from build123d import *

# Parameters (mm, degrees)
SKETCH1_W           = 609.6
SKETCH1_H           = 609.6
BOSS_EXTRUDE1_DEPTH = 6.35
CUT_EXTRUDE2_DEPTH  = 432.099063441
SKETCH4_W           = 25.4
SKETCH4_H           = 25.4
CUT_EXTRUDE8_DEPTH  = 432.099063441
FILLET4_R           = 12.7
FILLET5_R           = 12.7
SKETCH5_R           = 3.175
CUT_EXTRUDE9_DEPTH  = 432.099063441
FILLET9_R           = 1.5875


with BuildPart() as part:
    # Sketch1 → Boss-Extrude1 (new body)
    with BuildSketch(Plane(origin=(0, 0, 0), x_dir=(1, 0, 0), z_dir=(0, 1, 0))):
        Rectangle(SKETCH1_W, SKETCH1_H)
    extrude(amount=BOSS_EXTRUDE1_DEPTH)

    # Sketch3 → Cut-Extrude2 (cut, through all)
    with BuildSketch(Plane(origin=(0, 0, 0), x_dir=(1, 0, 0), z_dir=(0, 1, 0))):
        with BuildLine():
            Line((-3.175, 248.4755), (-3.175, 142.454689298))
            ThreePointArc((-3.175, 142.454689298), (-45.125573361, 120.304111538), (-50.492310608, 73.169232396))
            ThreePointArc((-50.492310608, 73.169232396), (-76.989658396, 44.45), (-88.612569335, 7.143007484))
            ThreePointArc((-88.612569335, 7.143007484), (-126.749203452, -21.072162878), (-124.95687982, -68.477713992))
            Line((-124.95687982, -68.477713992), (-216.773595218, -121.488119343))
            Line((-216.773595218, -121.488119343), (-213.598595218, -126.987380657))
            Line((-213.598595218, -126.987380657), (-121.78187982, -73.976975306))
            ThreePointArc((-121.78187982, -73.976975306), (-81.623630091, -99.23194866), (-38.120258727, -80.31223988))
            ThreePointArc((-38.120258727, -80.31223988), (0, -88.9), (38.120258727, -80.31223988))
            ThreePointArc((38.120258727, -80.31223988), (81.623630091, -99.23194866), (121.78187982, -73.976975306))
            Line((121.78187982, -73.976975306), (213.598595218, -126.987380657))
            Line((213.598595218, -126.987380657), (216.773595218, -121.488119343))
            Line((216.773595218, -121.488119343), (124.95687982, -68.477713992))
            ThreePointArc((124.95687982, -68.477713992), (126.749203452, -21.072162878), (88.612569335, 7.143007484))
            ThreePointArc((88.612569335, 7.143007484), (76.989658396, 44.45), (50.492310608, 73.169232396))
            ThreePointArc((50.492310608, 73.169232396), (45.125573361, 120.304111538), (3.175, 142.454689298))
            Line((3.175, 142.454689298), (3.175, 248.4755))
            Line((3.175, 248.4755), (-3.175, 248.4755))
        make_face()
    extrude(amount=CUT_EXTRUDE2_DEPTH, mode=Mode.SUBTRACT)

    # Sketch4 → Cut-Extrude8 (cut, through all)
    with BuildSketch(Plane(origin=(0, 0, 0), x_dir=(1, 0, 0), z_dir=(0, 1, 0))):
        with Locations((12.7, -190.5)):
            Rectangle(SKETCH4_W, SKETCH4_H)
        with Locations((-190.5, 12.7)):
            Rectangle(SKETCH4_W, SKETCH4_H)
    extrude(amount=CUT_EXTRUDE8_DEPTH, mode=Mode.SUBTRACT)

    # Fillet4
    fillet4_edges = [part.edges().sort_by_distance(p)[0] for p in [
        (-177.8, 3.175, -25.4),
    ]]
    fillet(fillet4_edges, radius=FILLET4_R)

    # Fillet5
    fillet5_edges = [part.edges().sort_by_distance(p)[0] for p in [
        (25.4, 3.175, 177.8),
    ]]
    fillet(fillet5_edges, radius=FILLET5_R)

    # Sketch5 → Cut-Extrude9 (cut, through all)
    with BuildSketch(Plane(origin=(0, 6.35, 0), x_dir=(1, 0, 0), z_dir=(0, 1, 0))):
        with Locations(Location((-254, 254, 0), (0, 0, 270))):
            Circle(SKETCH5_R)
        with Locations(Location((254, 254, 0), (0, 0, 270))):
            Circle(SKETCH5_R)
        with Locations(Location((254, -254, 0), (0, 0, 270))):
            Circle(SKETCH5_R)
        with Locations(Location((-254, -254, 0), (0, 0, 270))):
            Circle(SKETCH5_R)
    extrude(amount=-CUT_EXTRUDE9_DEPTH, mode=Mode.SUBTRACT)

    # Fillet9
    fillet9_edges = [part.edges().sort_by_distance(p)[0] for p in [
        (3.175, 3.175, -248.4755),
        (-3.175, 3.175, -248.4755),
        (-216.773595218, 3.175, 121.488119343),
        (-213.598595218, 3.175, 126.987380657),
        (213.598595218, 3.175, 126.987380657),
        (216.773595218, 3.175, 121.488119343),
    ]]
    fillet(fillet9_edges, radius=FILLET9_R)


solid = part.part
Check sheet for the modelled part. Datum: model origin and axes. Units: mm. A direction names the side the tool comes from. Round coordinates to 2 decimals unless told otherwise and drop trailing zeros. Loops run counter-clockwise (first coordinate to the right, second up) from the corner with the lowest first, then second, coordinate; pieces in that order, holes last. Notation, with made-up numbers: M 18,51 L 65,51 A33 cw 65,80 Z; hole C -40,40.25 d7. An arc over 180 degrees is marked long. One line per item, written item: value.
(1) Sectioned sample at A-A, the plane z = -66. Record the cut outline in (x, y), then the cut area to 3 significant figures.
Computed values:
outline: M -304.8,0 L -59.56,0 L -59.56,6.35 L -304.8,6.35 Z; M 59.56,0 L 304.8,0 L 304.8,6.35 L 59.56,6.35 Z
area: 3,110 mm^2
(2) Access from +Z, -Z, +X, -X, +Y, -Y to the whole of each face (thin tool, end or side, straight path). Record for faces 1 (the face through (166.37, 3.13, 99.72)), 2 (the face through (63, 6.35, -72)).
Computed values:
face 1: +Y, -Y
face 2: +Z, -Z, +X, -X, +Y
(3) Sectioned sample at B-B, the plane x = 106. Record the cut outline in (y, z).
Computed values:
outline: M 0,-304.8 L 6.35,-304.8 L 6.35,-1.12 L 0,-1.12 Z; M 0,90.82 L 6.35,90.82 L 6.35,304.8 L 0,304.8 Z
(4) Depth check by flat-ended pin: pin 1 Ø10 at (x, z) = (254, -254) entering from +Y. Enter the tip coordinate at first touch or a pass-through.
Computed values:
pin 1: stops at y = 6.35
(5) Release check for a two-part mould opening along Z. For faces 3 (the face through (-169.54, 3.13, 94.22)), 4 (the face through (63, 0, -72)) record: +Z half, -Z half, draft (parallel to the pull), parting line (faces both ways), or undercut.
Computed values:
face 3: undercut
face 4: draft
(6) Sectioned sample at C-C, the plane y = 4.25. Count the separate pieces of the cut face and the enclosed holes in it, then the cut area to 3 significant figures.
Computed values:
separate pieces: 1
enclosed holes: 7
area: 328,000 mm^2
(7) Thickness scan on line 1 (Z direction, x = -254, y = 4.75) (3 decimals); line 2 (X direction, y = 4, z = -256). Record the ranges inside material, lowest first.
Computed values:
line 1: z = -304.8 to -257.175, -250.825 to 250.825, 257.175 to 304.8
line 2: x = -304.8 to -256.47, -251.53 to 251.53, 256.47 to 304.8
